```python
from build123d import *

# Parameters (mm, degrees)
SKETCH1_R           = 7.25
SKETCH1_R_2         = 3.175
BOSS_EXTRUDE1_DEPTH = 30
SKETCH2_OUTSIDE_W   = 23.768
SKETCH2_OUTSIDE_H   = 23.768
SKETCH2_OUTSIDE_R   = 5.25
CUT_EXTRUDE1_DEPTH  = 10
SKETCH3_R           = 5.25
CUT_EXTRUDE2_DEPTH  = 10


with BuildPart() as part:
    # Sketch1 → Boss-Extrude1 (new body)
    with BuildSketch(Plane(origin=(0, 0, 0), x_dir=(1, 0, 0), z_dir=(0, 1, 0))):
        Circle(SKETCH1_R)
        Circle(SKETCH1_R_2, mode=Mode.SUBTRACT)
    extrude(amount=BOSS_EXTRUDE1_DEPTH)

    # Sketch2 outside → Cut-Extrude1 (cut)
    with BuildSketch(Plane(origin=(0, 30, 0), x_dir=(1, 0, 0), z_dir=(0, 1, 0))):
        Rectangle(SKETCH2_OUTSIDE_W, SKETCH2_OUTSIDE_H)
        Circle(SKETCH2_OUTSIDE_R, mode=Mode.SUBTRACT)
    extrude(amount=-CUT_EXTRUDE1_DEPTH, mode=Mode.SUBTRACT)

    # Sketch3 → Cut-Extrude2 (cut)
    with BuildSketch(Plane.XZ):
        Circle(SKETCH3_R)
    extrude(amount=-CUT_EXTRUDE2_DEPTH, mode=Mode.SUBTRACT)


solid = part.part
```
Read the model definition and answer for the solid it produces. Units are mm, in the model's axes. A direction names the side the tool comes from. Give positions to 0.01 mm unless a question says otherwise; leave off trailing zeros. Write each loop counter-clockwise with the first axis right and the second up, starting at its lowest first coordinate (ties: lowest second). Pieces come first, ordered by that corner, then holes. Notation, with made-up numbers: (8.5, -5) -> (14.5, -5) arc R25 cw to (14.5, 13) -> close; hole circle Ø8 at (44.5, 78). An arc over 180 degrees is marked (long way). Answer as a JSON object with one key per item and string values.
1) Section C-C on z = -3.5 is taken. Write down the section's boundary in (x, y).
Findings below:
{"outline": "(-6.35, 0) -> (-3.91, 0) -> (-3.91, 10) -> (3.91, 10) -> (3.91, 0) -> (6.35, 0) -> (6.35, 20) -> (3.91, 20) -> (3.91, 30) -> (-3.91, 30) -> (-3.91, 20) -> (-6.35, 20) -> close"}
2) Flat-ended cylindrical pins translate along their axes: pin 1 Ø7.5 at (x, z) = (0, 0) entering from -Y; pin 2 Ø1 at (x, y) = (1, 24.5) entering from +Z; pin 3 Ø1.5 at (x, y) = (-2.5, 14.5) entering from -Z. Find the tip coordinate at first contact, or state that the pin passes through.
Findings below:
{"pin 1": "stops at y = 10", "pin 2": "stops at z = 5.23", "pin 3": "stops at z = -7.04"}
3) Section D-D on x = -3.5 is taken. Write down the section's boundary in (y, z).
Findings below:
{"outline": "(0, -6.35) -> (20, -6.35) -> (20, -3.91) -> (30, -3.91) -> (30, 3.91) -> (20, 3.91) -> (20, 6.35) -> (0, 6.35) -> (0, 3.91) -> (10, 3.91) -> (10, -3.91) -> (0, -3.91) -> close"}
4) Straight lines are drawn through the part: probe 1 along X at (y, z) = (26.25, 0) (3 decimals); probe 2 along Z at (x, y) = (0, 5.5). For each, find the intervals that lie inside material, in ascending order. Write a range as from..to.
Findings below:
{"probe 1": "x = -5.25..-3.175, 3.175..5.25", "probe 2": "z = -7.25..-5.25, 5.25..7.25"}
5) For a pull along X with two mould halves and no side action, classify faces 1 (the cylindrical face through (5, 25.1, -1.6)), 2 (the flat face through (-0.1, 30, 3.4)), 3 (the cylindrical face through (5, 4.9, 1.6)) as pulls with the +X half, pulls with the -X half, needs draft (parallel to the pull), parting line crosses it, or undercut.
Findings below:
{"face 1": "parting line crosses it", "face 2": "needs draft", "face 3": "undercut"}
6) Section B-B on y = 11.25 is taken. Write down the section's boundary in (x, z) (3 decimals).
Findings below:
{"outline": "circle Ø14.5 at (0, 0); hole circle Ø6.35 at (0, 0)"}
7) A tool of negligible diameter and unlimited length cuts with its end or side. For faces 4 (the cylindrical face through (-0.69, 19.86, 3.1)), 5 (the flat face through (-0.1, 10, -3.4)), 6 (the flat face through (4, 20, -4)), from which of +Z, -Z, +X, -X, +Y, -Y can it reach the whole face along a straight path? Write none if from no direction.
Findings below:
{"face 4": "+Y, -Y", "face 5": "-Y", "face 6": "+Y"}
8) Section A-A on z = 0 is taken. Write down the section's boundary in (x, y) (3 decimals), then the cut area to 3 significant figures.
Findings below:
{"outline": "(-7.25, 0) -> (-5.25, 0) -> (-5.25, 10) -> (-3.175, 10) -> (-3.175, 30) -> (-5.25, 30) -> (-5.25, 20) -> (-7.25, 20) -> close; (3.175, 10) -> (5.25, 10) -> (5.25, 0) -> (7.25, 0) -> (7.25, 20) -> (5.25, 20) -> (5.25, 30) -> (3.175, 30) -> close", "area": "163 mm^2"}
